Geometry check sheet. Reference: drawing and pictorial views, mm from the part's lowest x, y, z. A direction names the side the tool comes from. Coordinates: 2 decimals unless noted, no trailing zeros. Write each loop counter-clockwise with the first axis right and the second up, starting at its lowest first coordinate (ties: lowest second). Pieces come first, ordered by that corner, then holes. Notation, with made-up numbers: (41.25, -10) -> (92.25, -10) arc R11 cw to (92.25, 4) -> close; hole circle Ø4 at (12, 82). An arc over 180 degrees is marked (long way). Use a Markdown table: item, result.
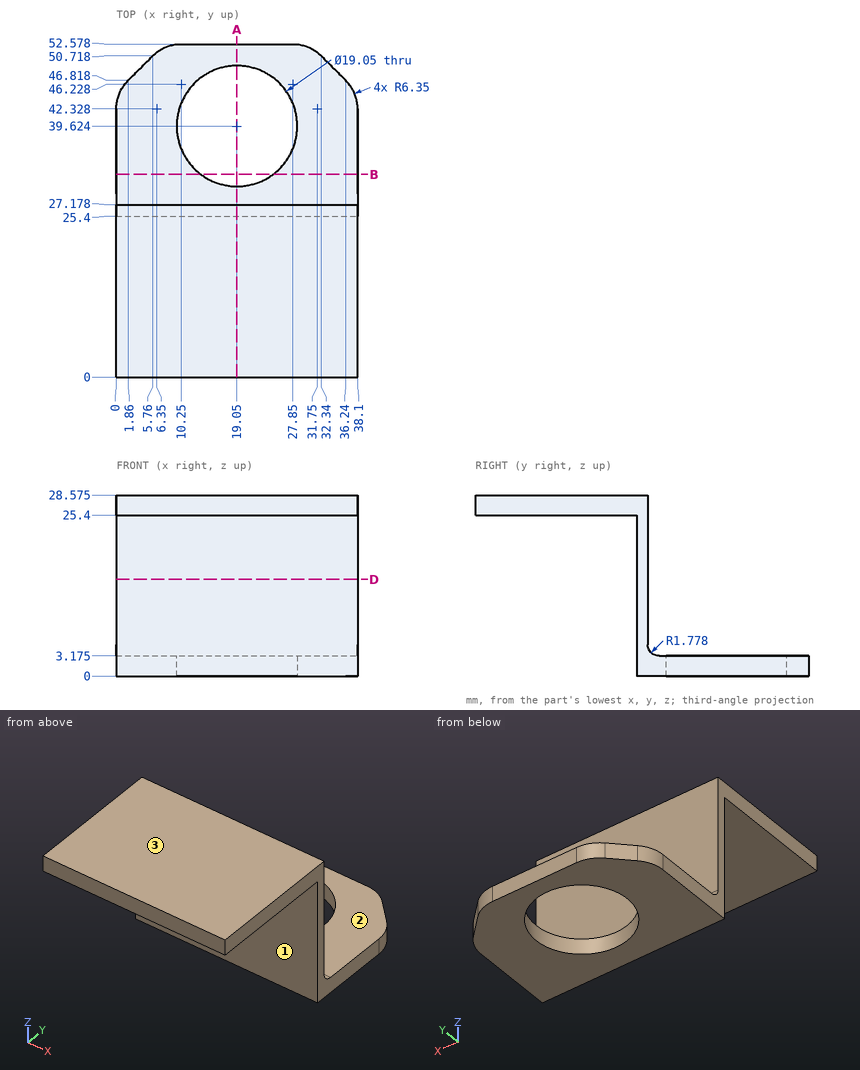
Item 1: Section check B-B on y = 32. Record the boundary of the cut face in (x, z) (1 decimal).
Answer block:
| item | result |
|---|---|
| outline | (0, 0) -> (13.3, 0) -> (13.3, 3.2) -> (0, 3.2) -> close; (24.8, 0) -> (38.1, 0) -> (38.1, 3.2) -> (24.8, 3.2) -> close |
Item 2: Depth check by flat-ended pin: P1, Ø12, axis at x = 18, y = 7, coming from the -Z side; P2, Ø5, axis at x = 8, z = 16, coming from the +Y side; P3, Ø4, axis at x = 28, z = 20.5, coming from the -Y side. Enter the tip coordinate at first touch or a pass-through.
Answer block:
| item | result |
|---|---|
| P1 | stops at z = 25.4 |
| P2 | stops at y = 27.18 |
| P3 | stops at y = 25.4 |
Item 3: Thickness scan on L1, parallel to Y at x = 19.05, z = 0.8; L2, parallel to Z at x = 25.5, y = 11 (1 decimal); L3, parallel to Z at x = 29, y = 47 (1 decimal). Record the ranges inside material, lowest first. Write a range as [from, to].
Answer block:
| item | result |
|---|---|
| L1 | y = [25.4, 30.1], [49.15, 52.58] |
| L2 | z = [25.4, 28.6] |
| L3 | z = [0, 3.2] |
Item 4: Section check D-D on z = 15.25. Record the boundary of the cut face in (x, y).
Answer block:
| item | result |
|---|---|
| outline | (0, 25.4) -> (38.1, 25.4) -> (38.1, 27.18) -> (0, 27.18) -> close |
Item 5: Section check A-A on x = 19.05. Record the boundary of the cut face in (y, z) (1 decimal).
Answer block:
| item | result |
|---|---|
| outline | (0, 25.4) -> (25.4, 25.4) -> (25.4, 0) -> (30.1, 0) -> (30.1, 3.2) -> (29, 3.2) arc R1.8 cw to (27.2, 5) -> (27.2, 28.6) -> (0, 28.6) -> close; (49.1, 0) -> (52.6, 0) -> (52.6, 3.2) -> (49.1, 3.2) -> close |
Item 6: Tool access check on the marked faces 1, 2 and 3. Record the directions out of +Z, -Z, +X, -X, +Y, -Y that give a thin tool (end or side, any length) a straight path to the whole face; none if there is none.
Answer block:
| item | result |
|---|---|
| face 1 | -Z, +X, -X, -Y |
| face 2 | +Z, +X, -X, +Y |
| face 3 | +Z, +X, -X, +Y, -Y |
